Job drawing, mm, ordinate dimensions from the low corner. One solid piece. A direction names the side the tool comes from. Give positions to 0.01 mm unless a question says otherwise; leave off trailing zeros. Write each loop counter-clockwise with the first axis right and the second up, starting at its lowest first coordinate (ties: lowest second). Pieces come first, ordered by that corner, then holes. Notation, with made-up numbers: M 60.25,75 L 108.25,75 A10 cw 108.25,94 Z; hole C -40,71.5 d8. An arc over 180 degrees is marked long. Answer as CSV lines item,"result". Start each with the question number.
1) Slice it at B-B, the plane z = 12.5. Give the cut face in (x, y), plus the area to 3 significant figures.
2) Slice it at C-C, the plane y = 25.5. Give the cut face in (x, z), plus the area to 3 significant figures.
3) Slice it at D-D, the plane y = 14.5. Give the cut face in (x, z), plus the area to 3 significant figures.
4) Pin check, flat tips, straight feed: pin 1 Ø6 at (x, y) = (19.5, 24.5) entering from +Z; pin 2 Ø7 at (x, z) = (12.5, 12.5) entering from +Y; pin 3 Ø6 at (x, y) = (6.5, 16) entering from -Z. Stop position of each tip, or through.
5) Mould opens along X. For the marked faces 3, 4 and 5 say: pulls with the +X half, pulls with the -X half, needs draft (parallel to the pull), parting line crosses it, or undercut.
6) Slice it at A-A, the plane x = 12.5. Give the cut face in (y, z), plus the area to 3 significant figures.
7) Tool access for the marked faces 1 and 2: list every direction of +Z, -Z, +X, -X, +Y, -Y with a clear straight run to the whole face (end or side of a thin tool).
8) Wall check: line 1 along Z through (x, y) = (12.5, 3.5); line 2 along Z through (x, y) = (12.5, 27); line 3 along X through (y, z) = (8.75, 13). Give the ranges that are in metal, low to high. Write a range as from..to.
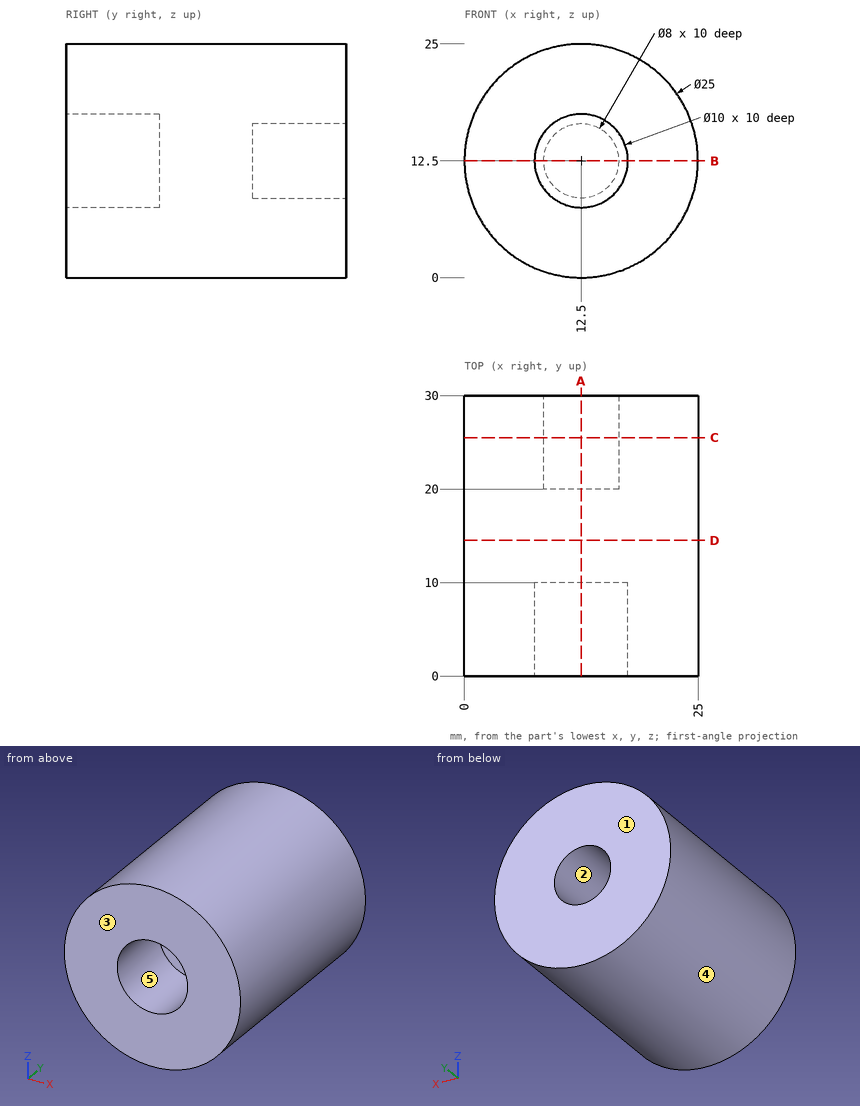
Found:
1,outline,"M 0,0 L 7.5,0 L 7.5,10 L 17.5,10 L 17.5,0 L 25,0 L 25,30 L 16.5,30 L 16.5,20 L 8.5,20 L 8.5,30 L 0,30 Z"
1,area,"570 mm²"
2,outline,"C 12.5,12.5 d25; hole C 12.5,12.5 d8"
2,area,"441 mm²"
3,outline,"C 12.5,12.5 d25"
3,area,"491 mm²"
4,pin 1,"z = 24.34"
4,pin 2,"y = 20"
4,pin 3,"z = 0.37"
5,face 3,"needs draft"
5,face 4,"parting line crosses it"
5,face 5,"undercut"
6,outline,"M 0,0 L 30,0 L 30,8.5 L 20,8.5 L 20,16.5 L 30,16.5 L 30,25 L 0,25 L 0,17.5 L 10,17.5 L 10,7.5 L 0,7.5 Z"
6,area,"570 mm²"
7,face 1,"+Z, -Z, +X, -X, +Y"
7,face 2,"+Y"
8,line 1,"0..7.5, 17.5..25"
8,line 2,"0..8.5, 16.5..25"
8,line 3,"0.01..7.53, 17.47..24.99"
